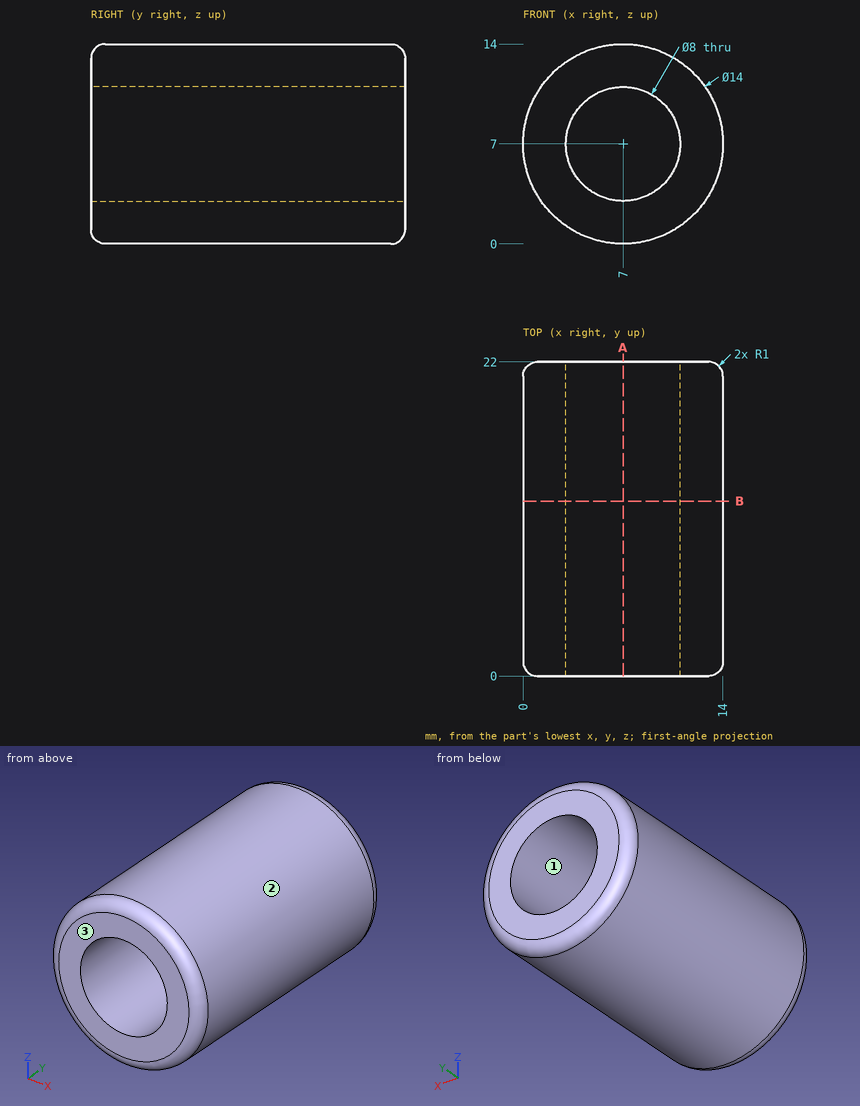
Verification items for this drawing (mm, ordinates from the low corner). Give positions to 0.01 mm unless a question says otherwise; leave off trailing zeros. Loops run counter-clockwise (first coordinate to the right, second up) from the corner with the lowest first, then second, coordinate; pieces in that order, holes last. Notation, with made-up numbers: M 28,-10.75 L 65,-10.75 A22 ccw 65,18.25 Z; hole C 76,72 d10. An arc over 180 degrees is marked long. Write each question's results on one line, items separated by ' | '.
1) Section check B-B, the plane y = 12.25. Record the boundary of the cut face in (x, z).
Answers follow:
outline: C 7,7 d14; hole C 7,7 d8
2) Section check A-A, the plane x = 7. Record the boundary of the cut face in (y, z), plus the area to 3 significant figures.
Answers follow:
outline: M 0,1 A1 ccw 1,0 L 21,0 A1 ccw 22,1 L 22,3 L 0,3 Z; M 0,11 L 22,11 L 22,13 A1 ccw 21,14 L 1,14 A1 ccw 0,13 Z | area: 131 mm2
3) Release check for a two-part mould opening along X. For the marked faces 1, 2 and 3 record: +X half, -X half, draft (parallel to the pull), parting line (faces both ways), or undercut.
Answers follow:
face 1: undercut | face 2: parting line | face 3: draft
4) Thickness scan on line 1 (X direction, y = 6.5, z = 7); line 2 (X direction, y = 7.5, z = 5.75); line 3 (Z direction, x = 9, y = 1.25). Record the ranges inside material, lowest first.
Answers follow:
line 1: 0 to 3, 11 to 14 | line 2: 0.11 to 3.2, 10.8 to 13.89 | line 3: 0.29 to 3.54, 10.46 to 13.71
5) Gauge pin test, flat end, axial feed: pin 1 (2 mm diameter, centred on x = 2.5, y = 6.5, fed in from -Z). Record the tip position at first contact, or that the pin passes through.
Answers follow:
pin 1: z = 0.94
